from build123d import *

# Parameters (mm, degrees)
SKETCH1_R           = 15
SKETCH1_R_2         = 7.5
BOSS_EXTRUDE1_DEPTH = 20
FILLET1_R           = 10
BOSS_EXTRUDE2_START = 10
SKETCH2_R           = 10
BOSS_EXTRUDE2_DEPTH = 80
SKETCH3_R           = 7.5
CUT_EXTRUDE1_DEPTH  = 40


with BuildPart() as part:
    # Sketch1 → Boss-Extrude1 (new body)
    with BuildSketch(Plane.XY):
        Circle(SKETCH1_R)
        Circle(SKETCH1_R_2, mode=Mode.SUBTRACT)
    extrude(amount=BOSS_EXTRUDE1_DEPTH)

    # Fillet1
    # the kernel refuses this fillet: 10 mm, written as the material it takes off along each edge
    with BuildSketch(Plane(origin=(0, 0, 0), x_dir=(1, 0, 0), z_dir=(0, -1, 0))) as fillet1_piece_1:
        with BuildLine():
            CenterArc((5, 9.682458366), FILLET1_R, 284.477512186, 75.522487814)
            Line((7.5, 0), (7.55, -0.193649167))
            ThreePointArc((7.55, -0.193649167), (11.25, -0.2), (15, -0.2))
            Line((15, -0.2), (15.2, 0))
            Line((15.2, 0), (15.2, 9.682458366))
            Line((15.2, 9.682458366), (15, 9.682458366))
        make_face()
    revolve(axis=Axis((0, 0, 0), (0, 0, 1)), mode=Mode.SUBTRACT)
    with BuildSketch(Plane(origin=(0, 0, 20), x_dir=(1, 0, 0), z_dir=(0, -1, 0))) as fillet1_piece_2:
        with BuildLine():
            CenterArc((5, -9.682458366), FILLET1_R, 0, 75.522487814)
            Line((7.5, 0), (7.55, 0.193649167))
            ThreePointArc((7.55, 0.193649167), (11.25, 0.2), (15, 0.2))
            Line((15, 0.2), (15.2, 0))
            Line((15.2, 0), (15.2, -9.682458366))
            Line((15.2, -9.682458366), (15, -9.682458366))
        make_face()
    revolve(axis=Axis((0, 0, 20), (0, 0, 1)), mode=Mode.SUBTRACT)

    # Sketch2 → Boss-Extrude2 (add)
    with BuildSketch(Plane(origin=(0, 0, 0), x_dir=(1, 0, 0), z_dir=(0, 1, 0)).offset(BOSS_EXTRUDE2_START)):
        with Locations(Location((0, -10, 0), (0, 0, 47.908263914))):
            Circle(SKETCH2_R)
    extrude(amount=BOSS_EXTRUDE2_DEPTH)

    # Sketch3 → Cut-Extrude1 (cut)
    with BuildSketch(Plane(origin=(0, 90, 0), x_dir=(1, 0, 0), z_dir=(0, 1, 0))):
        with Locations(Location((0, -10, 0), (0, 0, 270))):
            Circle(SKETCH3_R)
    extrude(amount=-CUT_EXTRUDE1_DEPTH, mode=Mode.SUBTRACT)


solid = part.part
Input: part model. Units: mm. Frame: model coordinates. Coordinates: 2 decimals unless noted, no trailing zeros. Order: outer loops, then holes, each group sorted by start corner. A loop starts at its lowest first (then second) coordinate and runs counter-clockwise, first axis right, second up. Notation, with made-up numbers: M -35,49.25 L 12,49.25 A32 cw 12,79.25 Z; hole C -35,68.25 d8. An arc over 180 degrees is marked long. Answer in a Markdown table with one row per item.
(1) Contact query for flat-ended pins moving along their axis: pin 1 Ø6 at (x, y) = (-5.5, 11) entering from +Z; pin 2 Ø1.3 at (x, z) = (2, 18) entering from -Y; pin 3 Ø1 at (x, z) = (0.5, 8) entering from -Y. Output: stop coordinate, or through.
Numbers:
| item | result |
|---|---|
| pin 1 | stops at z = 19.68 |
| pin 2 | stops at y = -11.95 |
| pin 3 | stops at y = -14.92 |
(2) Material intervals for line 1 (X direction, y = 66.5, z = 10); line 2 (Y direction, x = 0, z = 8); line 3 (Z direction, x = -4.5, y = 65), sorted ascending. Write a range as [from, to].
Numbers:
| item | result |
|---|---|
| line 1 | x = [-10, -7.5], [7.5, 10] |
| line 2 | y = [-14.86, -7.5], [7.5, 50] |
| line 3 | z = [1.07, 4], [16, 18.93] |
(3) Section query B-B, the plane y = 16.5. Output: boundary loops of the cut face in (x, z).
Numbers:
| item | result |
|---|---|
| outline | C 0,10 d20 |
(4) Section query A-A, the plane y = 69.5. Output: boundary loops of the cut face in (x, z).
Numbers:
| item | result |
|---|---|
| outline | C 0,10 d20; hole C 0,10 d15 |
(5) Draft query along Y for faces 1 (the cylindrical face through (-7.493, 0.33, 9.86)), 2 (the cylindrical face through (-0.51, -14.99, 10)), 3 (the flat face through (-5, 90, 4)). Return one class per face: pulls with the +Y half, pulls with the -Y half, needs draft (parallel to the pull), parting line crosses it, or undercut.
Numbers:
| item | result |
|---|---|
| face 1 | undercut |
| face 2 | parting line crosses it |
| face 3 | pulls with the +Y half |
